Can you work these out from the model? Positions are in its coordinate system, mm. A direction names the side the tool comes from. Give positions to 0.01 mm unless a question says otherwise; leave off trailing zeros. Loops run counter-clockwise (first coordinate to the right, second up) from the corner with the lowest first, then second, coordinate; pieces in that order, holes last. Notation, with made-up numbers: M 61.25,30 L 81.25,30 A17 cw 81.25,58 Z; hole C -32,-21.75 d1. An arc over 180 degrees is marked long. Answer as a JSON object with one key per item and string values.
```python
from build123d import *

# Parameters (mm, degrees)
SALIENTE_EXTRUIR1_DEPTH = 50
CROQUIS2_W              = 45
CROQUIS2_H              = 10
SALIENTE_EXTRUIR2_DEPTH = 20
CROQUIS3_W              = 45
CROQUIS3_H              = 10
SALIENTE_EXTRUIR3_DEPTH = 20


with BuildPart() as part:
    # Croquis1 → Saliente-Extruir1 (new body)
    with BuildSketch(Plane(origin=(0, 0, 0), x_dir=(0, 0, -1), z_dir=(1, 0, 0))):
        with BuildLine():
            Line((-54.179530832, 17.5), (245.820469168, 17.5))
            ThreePointArc((245.820469168, 17.5), (263.320469168, 0), (245.820469168, -17.5))
            Line((245.820469168, -17.5), (-54.179530832, -17.5))
            ThreePointArc((-54.179530832, -17.5), (-71.679530832, 0), (-54.179530832, 17.5))
        make_face()
        with BuildLine():
            Line((-54.179530832, 15), (245.820469168, 15))
            ThreePointArc((245.820469168, 15), (260.820469168, 0), (245.820469168, -15))
            Line((245.820469168, -15), (-54.179530832, -15))
            ThreePointArc((-54.179530832, -15), (-69.179530832, 0), (-54.179530832, 15))
        make_face(mode=Mode.SUBTRACT)
    extrude(amount=SALIENTE_EXTRUIR1_DEPTH)

    # Croquis2 → Saliente-Extruir2 (add)
    with BuildSketch(Plane(origin=(0, 17.5, 0), x_dir=(1, 0, 0), z_dir=(0, 1, 0))):
        with Locations((25, 190.820469168)):
            Rectangle(CROQUIS2_W, CROQUIS2_H)
        with Locations((25, 90.820469168)):
            Rectangle(CROQUIS2_W, CROQUIS2_H)
        with Locations((25, -9.179530832)):
            Rectangle(CROQUIS2_W, CROQUIS2_H)
    extrude(amount=SALIENTE_EXTRUIR2_DEPTH)

    # Croquis3 → Saliente-Extruir3 (add)
    with BuildSketch(Plane.XZ.offset(17.5)):
        with Locations((25, -190.820469168)):
            Rectangle(CROQUIS3_W, CROQUIS3_H)
        with Locations((25, -90.820469168)):
            Rectangle(CROQUIS3_W, CROQUIS3_H)
        with Locations((25, 9.179530832)):
            Rectangle(CROQUIS3_W, CROQUIS3_H)
    extrude(amount=SALIENTE_EXTRUIR3_DEPTH)


solid = part.part
```
1) Suppose I cut it at B-B, the plane y = 0. Write out the boundary of the cut face in (x, z).
Answer list:
{"outline": "M 0,-263.32 L 50,-263.32 L 50,-260.82 L 0,-260.82 Z; M 0,69.18 L 50,69.18 L 50,71.68 L 0,71.68 Z"}
2) Suppose I cut it at A-A, the plane z = -177.5. Write out the boundary of the cut face in (x, y).
Answer list:
{"outline": "M 0,-17.5 L 50,-17.5 L 50,-15 L 0,-15 Z; M 0,15 L 50,15 L 50,17.5 L 0,17.5 Z"}
3) Will these pins go through, and if not, where does the flat tip stop? pin 1 Ø3 at (y, z) = (27, -89.5) entering from +X; pin 2 Ø2 at (x, z) = (15, -105.5) entering from +Y; pin 3 Ø16 at (x, y) = (14, -28.5) entering from -Z.
Answer list:
{"pin 1": "x = 47.5", "pin 2": "y = 17.5", "pin 3": "z = -195.82"}
4) Please list where these lines run through material, in increasing order: line 1 along Z through (x, y) = (8.5, -25.5); line 2 along Y through (x, z) = (46.5, -50); line 3 along Z through (x, y) = (33, -1). Write a range as from..to.
Answer list:
{"line 1": "-195.82..-185.82, -95.82..-85.82, 4.18..14.18", "line 2": "-17.5..-15, 15..17.5", "line 3": "-263.29..-260.79, 69.15..71.65"}
5) If we mould it in two halves opening along Y, with no side actions, what happens to faces 1 (the flat face through (2.5, 27, -91)), 2 (the flat face through (25, 37.5, -191)), 3 (the cylindrical face through (24.65, -0.33, 69.176))? For each: +Y half, -Y half, draft (parallel to the pull), parting line (faces both ways), or undercut.
Answer list:
{"face 1": "draft", "face 2": "+Y half", "face 3": "undercut"}
6) For faces 4 (the flat face through (25, 27, 4.18)), 5 (the flat face through (2.5, -27, -91)), 6 (the flat face through (47.5, 27, -191)), 7 (the flat face through (25, -27, -85.82)), 8 (the flat face through (47.5, -27, 9)), which set-ups out of +Z, -Z, +X, -X, +Y, -Y let a thin tool reach every point of the face, with its end or its side?
Answer list:
{"face 4": "+X, -X, +Y", "face 5": "+Z, -Z, -X, -Y", "face 6": "+Z, -Z, +X, +Y", "face 7": "+X, -X, -Y", "face 8": "+Z, -Z, +X, -Y"}
